Autodesk Inventor part; units mm, degrees
ref_plane "YZ Plane" through (0, 0, 0) normal (1, 0, 0) x (0, 1, 0)
ref_plane "XZ Plane" through (0, 0, 0) normal (0, 1, 0) x (-1, 0, 0)
ref_plane "XY Plane" through (0, 0, 0) normal (0, 0, 1) x (1, 0, 0)
sketch "Sketch1" plane through (0, 0, 0) normal (0, 1, 0) x (-1, 0, 0)
  arc A0 (-2.54, 0) -> (0, 2.54) centre (0, 0) ccw
  line L0 (0, 2.54) -> (0, 0)
  line L1 (0, 0) -> (-2.54, 0)
  dimension "d0" = 5.08
extrude "Extrusion1" add sketch "Sketch1" along normal blind 25.4
sketch "Sketch2" plane through (0, 25.4, 0) normal (0, 1, 0) x (1, 0, 0)
  line L0 (0, -2.54) -> (0, 0)
  line L1 (0, 0) -> (-17.9605, 17.9605)
  line L2 (0, 0) -> (25.4, 0) construction
  line L3 (0, 0) -> (-1.7961, -1.7961)
  arc A0 (2.54, 0) -> (0, -2.54) centre (0, 0) ccw
  line L4 (0, 0) -> (1.7961, 1.7961)
  line L5 (-1.7961, -1.7961) -> (-19.7566, 16.1645)
  line L6 (-19.7566, 16.1645) -> (-17.9605, 17.9605)
  line L7 (-16.1645, 19.7566) -> (1.7961, 1.7961)
  line L8 (-16.1645, 19.7566) -> (-17.9605, 17.9605)
  line L9 (0, 0) -> (2.54, 0)
  dimension "d3" = 25.4
  dimension "d4" = 135
extrude "Extrusion2" add sketch "Sketch2" along normal blind 6
sketch "Sketch3" plane through (-19.7566, 25.4, -16.1645) normal (-0.7071068, 0, -0.7071068) x (-0.7071068, 0, 0.7071068)
  line L0 (-5.08, 0) -> (-5.08, 6)
  line L1 (0, 6) -> (-5.08, 6)
  line L2 (-5.08, 6) -> (-5.08, 0)
  line L3 (-5.08, 0) -> (0, 0)
  line L4 (0, 0.5) -> (0, 5.5)
  line L5 (-2.54, 6) -> (-4.3361, 6)
  line L6 (-2.54, 6) -> (-2.54, 0)
  line L7 (-4.54, 0) -> (-0.54, 0)
  line L8 (-0.54, 0.5) -> (-0.54, 5.5)
  line L9 (-0.54, 6) -> (-4.54, 6)
  line L10 (-4.54, 6) -> (-4.54, 0)
  line L11 (-4.54, 0) -> (-0.54, 6) construction
  line L12 (-0.54, 0) -> (-4.54, 6) construction
  line L13 (0, 0.5) -> (-5.08, 0.5)
  line L14 (-5.08, 0.5) -> (-5.08, 5.5)
  line L15 (-5.08, 5.5) -> (0, 5.5)
  line L16 (0, 0.5) -> (-5.08, 5.5) construction
  line L17 (-5.08, 0.5) -> (0, 5.5) construction
  line L18 (-5.08, 0) -> (0, 0)
  line L19 (0, 0) -> (0, 6)
  line L20 (0, 6) -> (-5.08, 6)
  line L21 (-5.08, 6) -> (-5.08, 0)
  line L22 (-5.08, 0) -> (0, 6) construction
  line L23 (0, 0) -> (-5.08, 6) construction
  line L24 (-0.7439, 6) -> (0, 6)
  line L25 (-5.08, 0) -> (0, 0)
  line L26 (0, 0) -> (0, 6)
  line L27 (0, 6) -> (-5.08, 6)
  line L28 (-5.08, 6) -> (-5.08, 0)
  line L29 (-5.08, 0) -> (0, 6) construction
  line L30 (0, 0) -> (-5.08, 6) construction
  line L31 (0, 6) -> (0, 0)
  line L32 (-4.54, 5.5) -> (-9.54, 5.5)
  line L33 (-9.54, 5.5) -> (-9.54, 0.5)
  line L34 (-9.54, 0.5) -> (-4.54, 0.5)
  line L35 (-4.54, 0.5) -> (-4.54, 5.5)
  line L36 (-0.54, 5.5) -> (4.46, 5.5)
  line L37 (4.46, 5.5) -> (4.46, 0.5)
  line L38 (4.46, 0.5) -> (-0.54, 0.5)
  line L39 (-0.54, 0.5) -> (-0.54, 5.5)
  point P0 (-2.54, -25.4)
  point P1 (-2.54, 3)
  point P2 (-4.54, 5.5)
  point P3 (-5.08, 5.5)
  point P4 (-5.08, 0.5)
  point P5 (-4.54, 0.5)
  point P6 (0, 5.5)
  point P7 (0, 0.5)
  point P8 (-5.08, 0.5)
  point P9 (-5.08, 5.5)
  dimension "d7" = 4
  dimension "d8" = 5
  dimension "d11" = 6
  dimension "d40" = 5
  dimension "d41" = 5
extrude "Extrusion5" cut sketch "Sketch3" against normal blind 33.8125 contours L34 L33 L32 L0 | L0 L15 L10 L13 | L8 L15 L4 L13 | L4 L36 L37 L38
sketch "Sketch6" plane through (0, 31.4, 0) normal (0, 1, 0) x (1, 0, 0)
  arc A0 (1.7961, 1.7961) -> (-1.7961, -1.7961) centre (0, 0) ccw
  circle A1 centre (0, 0) radius 2.54
  line L0 (1.7961, 1.7961) -> (-16.1645, 19.7566)
  line L1 (0, 3.5921) -> (-3.5921, 0)
  line L2 (-19.7566, 16.1645) -> (-1.7961, -1.7961)
  line L3 (-1.7961, 1.7961) -> (-2.5032, 2.5032)
  circle A2 centre (-2.5032, 2.5032) radius 2.54
  dimension "d16" = 1
ref_plane "Work Plane3" through (-2.5032, 37.9, -2.5032) normal (0, 1, 0) x (1, 0, 0)
sketch "Sketch7" plane through (-2.5032, 37.9, -2.5032) normal (0, 1, 0) x (1, 0, 0)
  circle A0 centre (0, 0) radius 1.5
  point P0 (2.5032, -2.5032)
  dimension "d19" = 3
extrude "Extrusion7" cut sketch "Sketch7" against normal blind 6
sketch "Sketch10" plane through (0, 31.4, 0) normal (0, 1, 0) x (1, 0, 0)
  arc A0 (-1.7961, -1.7961) -> (0, -2.54) centre (0, 0) ccw
  line L0 (0, -2.54) -> (0, 0)
  line L1 (0, 0) -> (2.54, 0)
  line L2 (1.7961, 1.7961) -> (-16.1645, 19.7566)
  line L3 (-19.7566, 16.1645) -> (-1.7961, -1.7961)
  line L4 (-19.7566, 16.1645) -> (-1.7961, -1.7961)
  line L5 (-16.1645, 19.7566) -> (-19.7566, 16.1645)
  line L6 (1.7961, 1.7961) -> (-16.1645, 19.7566)
  arc A1 (2.54, 0) -> (1.7961, 1.7961) centre (0, 0) ccw
  point P0 (-0.7071, 4.2992)
  point P1 (2.5214, 0.3071)
  point P2 (-4.2992, 0.7071)
extrude "Extrusion9" add sketch "Sketch10" along normal blind 1.5
sketch "Sketch11" plane through (0, 25.4, 0) normal (0, -1, 0) x (1, 0, 0)
  arc A0 (-1.7961, 1.7961) -> (1.7961, -1.7961) centre (0, 0) ccw
  line L0 (-19.7566, -16.1645) -> (-1.7961, 1.7961)
  line L1 (-16.1645, -19.7566) -> (-19.7566, -16.1645)
  line L2 (1.7961, -1.7961) -> (-16.1645, -19.7566)
extrude "Extrusion10" add sketch "Sketch11" along normal blind 1.5
sketch "Sketch13" plane through (0, 0, 0) normal (0, -1, 0) x (1, 0, 0)
  line L0 (0, 0) -> (2.54, 0)
  arc A0 (0, 5) -> (5, 0) centre (0, 0) ccw
  line L1 (0, 0) -> (0, 5)
  line L2 (0, 0) -> (5, 0)
  dimension "d37" = 10
extrude "Extrusion12" add sketch "Sketch13" against normal up to surface (23.9 mm away)
sketch "Sketch14" plane through (0, 0, 0) normal (0, -1, 0) x (1, 0, 0)
  circle A0 centre (0, 0) radius 1
  dimension "d42" = 2
extrude "Extrusion13" cut sketch "Sketch14" against normal blind 11.2
sketch "Sketch15" plane through (0, 32.9, 0) normal (0, 1, 0) x (1, 0, 0)
  circle A0 centre (-2.5032, 2.5032) radius 1.5
  circle A1 centre (-2.5032, 2.5032) radius 1.5
  point P0 (0, 0)
extrude "Extrusion14" cut sketch "Sketch15" against normal blind 8
thread "Thread2"
sketch "Sketch16" plane through (0, 0, 0) normal (0, -1, 0) x (1, 0, 0)
  arc A0 (0, 5) -> (5, 0) centre (0, 0) ccw
  line L0 (0, 0) -> (3.981, 3.981)
  line L1 (0, 0) -> (5.63, 0) construction
  line L2 (0, 5) -> (-5, 0)
  line L3 (5, 0) -> (0, -5)
  line L4 (-5, 0) -> (0, -5)
  circle A1 centre (0, 0) radius 5
  dimension "d52" = 45
extrude "Extrusion15" cut sketch "Sketch16" against normal up to surface (23.9 mm away) contours L2 A0 | L4 A0 | L3 A0
sketch "Sketch17" plane through (-19.3747, 25.9, -16.5463) normal (-0.7071068, 0, -0.7071068) x (-0.7071068, 0, 0.7071068)
  line L0 (0, 0) -> (0.54, 0)
  line L1 (0.54, 5) -> (0, 5)
  line L2 (-4, 0) -> (-4, 5)
  line L3 (-4.54, 0) -> (-4, 0)
  line L4 (-4, 5) -> (-4.54, 5)
  line L5 (0.54, -2) -> (0.54, 0)
  line L6 (0.54, -2) -> (-0.2039, -2)
  line L7 (-2, 7) -> (-3.7961, 7)
  line L8 (-4.54, 5) -> (-4.54, 7)
  line L9 (-3.7961, 7) -> (-4.54, 7)
  line L10 (0.54, -2) -> (-0.2039, -2)
  line L11 (-0.2039, -2) -> (-0.2039, 7)
  line L12 (0.54, 7) -> (-0.2039, 7)
  line L13 (0.54, 5) -> (0.54, 7)
  line L14 (0.54, 5) -> (0, 5)
  line L15 (0, 5) -> (0, 0)
  line L16 (0, 0) -> (0.54, 0)
  line L17 (0.54, -2) -> (0.54, 0)
  line L18 (-3.7961, -2) -> (-3.7961, 7)
  line L19 (-3.7961, -2) -> (-4.54, -2)
  line L20 (-4.54, -2) -> (-4.54, 0)
  line L21 (-4.54, 0) -> (-4, 0)
  line L22 (-4, 0) -> (-4, 5)
  line L23 (-4, 5) -> (-4.54, 5)
  line L24 (-4.54, 5) -> (-4.54, 7)
  line L25 (-3.7961, 7) -> (-4.54, 7)
  line L26 (-3.7961, -2) -> (-3.7961, 7)
  line L27 (0.54, -2) -> (-4.54, -2)
  line L28 (0, 5) -> (0, 0)
  line L29 (-3.7961, -2) -> (-4.54, -2)
  line L30 (0.54, -2) -> (-4.54, -2)
  line L31 (0.54, 0) -> (0, 0)
  line L32 (0, 0) -> (0, 5)
  line L33 (0, 5) -> (0.54, 5)
  line L34 (0.54, 5) -> (0.54, 7)
  line L35 (-4.54, 7) -> (0.54, 7)
  line L36 (-4.54, 5) -> (-4.54, 7)
  line L37 (-4.54, 5) -> (-4, 5)
  line L38 (-4, 5) -> (-4, 0)
  line L39 (-4, 0) -> (-4.54, 0)
  line L40 (-4.54, -2) -> (-4.54, 0)
  line L41 (0.54, -2) -> (-4.54, -2)
  line L42 (0.54, 0) -> (0.54, -2)
  line L43 (-3.5, 7) -> (-0.5, 7)
  line L44 (-0.2039, 7) -> (-2, 7)
  line L45 (-2, 7) -> (-3.7961, 7)
  line L46 (-3.7961, 7) -> (-4.54, 7)
  line L47 (-4.54, 7) -> (0.54, 7)
  line L48 (0.54, 7) -> (-0.2039, 7)
  line L49 (0.54, -2) -> (-4.54, -2)
  line L50 (0.54, -2) -> (-4.54, -2)
  line L51 (0.54, 5) -> (0.54, 7)
  line L52 (0, 5) -> (0.54, 5)
  line L53 (0.54, 5) -> (0.54, 7)
  line L54 (0.54, 0) -> (0, 0)
  line L55 (0.54, 5) -> (0.54, 7)
  line L56 (0.54, 5) -> (0.54, 7)
  line L57 (0.54, 0) -> (0.54, -2)
  line L58 (0.54, -2) -> (0.54, 0)
  line L59 (0.54, 5) -> (0, 5)
  line L60 (0, 5) -> (0.54, 5)
  line L61 (0, 0) -> (0.54, 0)
  line L62 (0.54, 0) -> (0, 0)
  line L63 (0, 5) -> (0, 0)
  line L64 (0, 0) -> (0, 5)
  line L65 (-4.54, -2) -> (-4.54, 0)
  line L66 (0.54, 7) -> (-0.2039, 7)
  line L67 (-4.54, 5) -> (-4.54, 7)
  line L68 (-4.54, -2) -> (-4.54, 0)
  line L69 (-4, 0) -> (-4.54, 0)
  line L70 (-4.54, 5) -> (-4, 5)
  line L71 (-4, 0) -> (-4, 5)
  line L72 (-4, 5) -> (-4, 0)
  line L73 (-4, 0) -> (-4.54, 0)
  line L74 (-4.54, 0) -> (-4, 0)
  line L75 (-4, 5) -> (-4.54, 5)
  line L76 (-4.54, 5) -> (-4, 5)
  line L77 (-4.54, -2) -> (-4.54, 0)
  line L78 (-4.54, -2) -> (-4.54, 0)
  line L79 (-4.54, 5) -> (-4.54, 7)
  line L80 (-4.54, 5) -> (-4.54, 7)
  line L81 (-4.54, 7) -> (0.54, 7)
  line L82 (-4, 5) -> (-4, 0)
  line L83 (0.54, 0) -> (0.54, -2)
  line L84 (-0.2039, -2) -> (-0.2039, 7)
  line L85 (-3.5, -1) -> (-0.5, -1)
  line L86 (-3.5, -1) -> (-0.5, -1)
  line L87 (-3.5, 7) -> (-0.5, 7)
  line L88 (-3.5, -1) -> (-0.5, -1)
  line L89 (-3.5, 7) -> (-0.5, 7)
  line L90 (0, 0) -> (0, 5)
  line L91 (-0.2039, 7) -> (-2, 7)
  line L92 (0.54, 5.5) -> (-4.54, 5.5)
  line L93 (0.54, 5.5) -> (-4.54, 5.5)
  line L94 (-4.54, 5.5) -> (0.54, 5.5)
  line L95 (0.54, 5.5) -> (-4.54, 5.5)
  point P0 (-2, -25.9)
  point P1 (-2, 5.5)
  point P2 (-2, 5.5)
  point P3 (-2, 5.5)
  point P4 (-4.54, 5.5)
  point P5 (0.54, 5.5)
  point P6 (0.54, 5.5)
  point P7 (-2, 5.5)
  point P8 (-2, 5.5)
  point P9 (-2, 5.5)
  point P10 (-2, 5.5)
sketch "Sketch18" plane through (0, 32.9, 0) normal (0, 1, 0) x (1, 0, 0)
  point P0 (0, 0)
sketch "Sketch19" plane through (0, 0, 0) normal (0, -1, 0) x (1, 0, 0)
  arc A0 (-0.3071, 2.5214) -> (-1.7961, 1.7961) centre (0, 0) ccw
  arc A1 (-0.3071, 2.5214) -> (-1.7961, 1.7961) centre (0, 0) ccw
  arc A2 (1.7961, -1.7961) -> (2.5214, -0.3071) centre (0, 0) ccw
  arc A3 (1.7961, -1.7961) -> (2.5214, -0.3071) centre (0, 0) ccw
  arc A4 (0, 2.54) -> (-1.7961, 1.7961) centre (0, 0) ccw
  line L0 (0, 5) -> (0, 2.54)
  line L1 (0, 0) -> (2.54, 0)
  line L2 (-1.7961, 1.7961) -> (-4.2961, -0.7039)
  arc A5 (1.7961, -1.7961) -> (2.54, 0) centre (0, 0) ccw
  line L3 (-4.2961, -0.7039) -> (-5, 0)
  arc A6 (0, 2.54) -> (-1.7961, 1.7961) centre (0, 0) ccw
  arc A7 (0, 2.54) -> (-1.7961, 1.7961) centre (0, 0) ccw
  arc A8 (-0.3071, 2.5214) -> (-1.7961, 1.7961) centre (0, 0) ccw
  arc A9 (-0.3071, 2.5214) -> (-1.7961, 1.7961) centre (0, 0) ccw
  line L4 (-5, 0) -> (0, 5)
  line L5 (-5, 0) -> (0, 5)
  line L6 (0, 5) -> (0, 2.54)
  arc A10 (0, 2.54) -> (-1.7961, 1.7961) centre (0, 0) ccw
  line L7 (-1.7961, 1.7961) -> (-4.2961, -0.7039)
  line L8 (-4.2961, -0.7039) -> (-5, 0)
  arc A11 (1.7961, -1.7961) -> (2.54, 0) centre (0, 0) ccw
  arc A12 (1.7961, -1.7961) -> (2.5214, -0.3071) centre (0, 0) ccw
  arc A13 (1.7961, -1.7961) -> (2.5214, -0.3071) centre (0, 0) ccw
  arc A14 (1.7961, -1.7961) -> (2.54, 0) centre (0, 0) ccw
  line L9 (-4.2961, -0.7039) -> (-0.7039, -4.2961)
  line L10 (0, 1) -> (0, 0)
  line L11 (0, 1) -> (0, 0)
  line L12 (0, 2.54) -> (0, 0)
  line L13 (0, 5) -> (0, 2.54)
  line L14 (0, 5) -> (0, 1)
  line L15 (0, 0) -> (1, 0)
  line L16 (1, 0) -> (5, 0)
  line L17 (2.54, 0) -> (5, 0)
  line L18 (0, 0) -> (2.54, 0)
  line L19 (5, 0) -> (0, -5)
  line L20 (0, -5) -> (5, 0)
  line L21 (-4.2961, -0.7039) -> (-5, 0)
  line L22 (-4.2961, -0.7039) -> (-0.7039, -4.2961)
  line L23 (0, -5) -> (-0.7039, -4.2961)
  line L24 (-5, 0) -> (0, -5)
  line L25 (-5, 0) -> (0, -5)
  line L26 (0, 5) -> (-5, 0)
  line L27 (-5, 0) -> (0, 5)
  line L28 (0, 5) -> (-5, 0)
  line L29 (0, -5) -> (-0.7039, -4.2961)
  arc A15 (1.7961, -1.7961) -> (2.54, 0) centre (0, 0) ccw
  line L30 (-0.7039, -4.2961) -> (1.7961, -1.7961)
  line L31 (2.54, 0) -> (5, 0)
  line L32 (5, 0) -> (0, -5)
  line L33 (0, -5) -> (-0.7039, -4.2961)
  line L34 (-0.7039, -4.2961) -> (1.7961, -1.7961)
  arc A16 (1.7961, -1.7961) -> (2.54, 0) centre (0, 0) ccw
  line L35 (2.54, 0) -> (5, 0)
  line L36 (5, 0) -> (0, -5)
  arc A17 (0, 2.54) -> (-1.7961, 1.7961) centre (0, 0) ccw
  circle A18 centre (-2.5032, -2.5032) radius 1.5
  circle A19 centre (-2.5032, -2.5032) radius 1.5
  circle A20 centre (-2.5032, -2.5032) radius 1.5
  circle A21 centre (-2.5032, -2.5032) radius 1.5
  circle A22 centre (-2.5032, -2.5032) radius 1.5
  line L37 (0, 5) -> (0, 1)
  arc A23 (0, 1) -> (1, 0) centre (0, 0) ccw
  line L38 (0, -5) -> (5, 0)
  line L39 (1, 0) -> (5, 0)
  line L40 (0, 0) -> (1, 0)
  arc A24 (0, 1) -> (1, 0) centre (0, 0) ccw
  line L41 (0, 0) -> (1, 0)
  line L42 (0, 1) -> (0, 0)
  arc A25 (0, 1) -> (1, 0) centre (0, 0) ccw
  arc A26 (0, 1) -> (1, 0) centre (0, 0) ccw
  arc A27 (0, 1) -> (1, 0) centre (0, 0) ccw
  line L43 (0, 5) -> (-5, 0)
  line L44 (-5, 0) -> (0, -5)
  line L45 (0, -5) -> (5, 0)
  line L46 (1, 0) -> (5, 0)
  arc A28 (0, 1) -> (1, 0) centre (0, 0) ccw
  line L47 (0, 5) -> (0, 1)
  line L48 (0, 2.54) -> (0, 0)
  arc A29 (-1.7961, 1.7961) -> (1.7961, -1.7961) centre (0, 0) ccw
  circle A30 centre (0, 0) radius 2.54
  line L49 (0, -3.5921) -> (-3.5921, 0)
  line L50 (-1.7961, -1.7961) -> (-2.5032, -2.5032)
  circle A31 centre (-2.5032, -2.5032) radius 2.54
  line L51 (-19.7566, -16.1645) -> (-16.1645, -19.7566)
  dimension "d55" = 21.8645
properties part number "Redesign_Gripper_Finger_3DPrint"
Geometry check sheet. Reference: the model listing, model coordinates, mm. A direction names the side the tool comes from. Coordinates: 2 decimals unless noted, no trailing zeros. Order: outer loops, then holes, each group sorted by start corner. A loop starts at its lowest first (then second) coordinate and runs counter-clockwise, first axis right, second up.
Item 1: Section check A-A (y = 7). Enter the section's corners in (x, z).
Item 2: Mould release check, pull along Y, two halves, no side actions. Record for faces 1 (the flat face through (-7, 30.9, -10.2)), 2 (the flat face through (2, 23.9, -2)), 3 (the flat face through (-1, 0, -1)): released by +Y, released by -Y, zero draft, split by the parting line, or undercut.
Item 3: Scan lines: line 1 along Y through (x, z) = (-2, -5); line 2 along Y through (x, z) = (-14.25, -13.75); line 3 along Z through (x, y) = (-3.5, 29.5). Record each from-to range of solid material in increasing order.
Item 4: Tool access check on faces 4 (the flat face through (-2, 23.9, 2)), 5 (the cylindrical face through (2.341, 32.14, -0.985)), 6 (the flat face through (0, 16, 3)), 7 (the flat face through (-10.2, 30.9, -7)). Record the directions out of +Z, -Z, +X, -X, +Y, -Y that give a thin tool (end or side, any length) a straight path to the whole face; none if there is none.
Item 5: Section check B-B (z = -3.25). Enter the section's corners in (x, y), plus the area to 3 significant figures.
Item 6: Section check D-D (y = 15). Enter the section's corners in (x, z), plus the area to 3 significant figures.
Item 7: Depth check by flat-ended pin: pin 1 (2.5 mm diameter, centred on y = 13.5, z = 3, fed in from +X); pin 2 (1.5 mm diameter, centred on y = 15, z = -3.5, fed in from +X); pin 3 (8 mm diameter, centred on x = -11.5, z = -3.5, fed in from -Y); pin 4 (3 mm diameter, centred on x = -4, z = -11, fed in from -Y). Enter the tip coordinate at first touch or a pass-through.
Item 8: Section check C-C (x = -14.25). Enter the section's corners in (y, z), plus the area to 3 significant figures.
Check sheet entries:
1. outline: (-5, 0) - (0, -5) - (5, 0) - (1, 0) arc R1 cw (long way) to (0, 1) - (0, 5) - close
2. face 1: undercut
2. face 2: released by +Y
2. face 3: released by -Y
3. line 1: y = 23.9 to 25.9, 30.9 to 32.9
3. line 2: y = 23.9 to 32.9
3. line 3: z = -6.33 to -3.62, -1.38 to -0.67
4. face 4: +Z, -X, +Y
4. face 5: -Z, +X, +Y
4. face 6: +Z, +X, +Y, -Y
4. face 7: +Z, -X
5. outline: (-6.84, 23.9) - (-1.75, 23.9) - (-1.75, 0) - (1.75, 0) - (1.75, 23.9) - (0.34, 23.9) - (0.34, 25.9) - (-0.42, 25.9) - (-0.42, 30.9) - (0.34, 30.9) - (0.34, 32.9) - (-1.2, 32.9) - (-1.2, 24.9) - (-3.8, 24.9) - (-3.8, 32.9) - (-6.84, 32.9) - (-6.84, 30.9) - (-6.08, 30.9) - (-6.08, 25.9) - (-6.84, 25.9) - close
5. area: 120 mm2
6. outline: (-5, 0) - (0, -5) - (5, 0) - (0, 0) - (0, 5) - close
6. area: 37.5 mm2
7. pin 1: stops at x = 0
7. pin 2: stops at x = 2.25
7. pin 3: stops at y = 23.9
7. pin 4: passes through
8. outline: (23.9, -17.84) - (25.9, -17.84) - (25.9, -17.08) - (30.9, -17.08) - (30.9, -17.84) - (32.9, -17.84) - (32.9, -10.66) - (30.9, -10.66) - (30.9, -11.42) - (25.9, -11.42) - (25.9, -10.66) - (23.9, -10.66) - close
8. area: 57.0 mm2
